Geometry: see drawing. Coordinates: mm, zero at the bounding-box minimum. Coordinates: 2 decimals unless noted, no trailing zeros. Loops run counter-clockwise (first coordinate to the right, second up) from the corner with the lowest first, then second, coordinate; pieces in that order, holes last. Notation, with made-up numbers: (-15.75, 59.5) -> (32.25, 59.5) arc R20 cw to (32.25, 63.5) -> close; hole circle Ø2 at (-10, -31.5). An arc over 180 degrees is marked (long way). Answer as a JSON object with one key per item and string values.
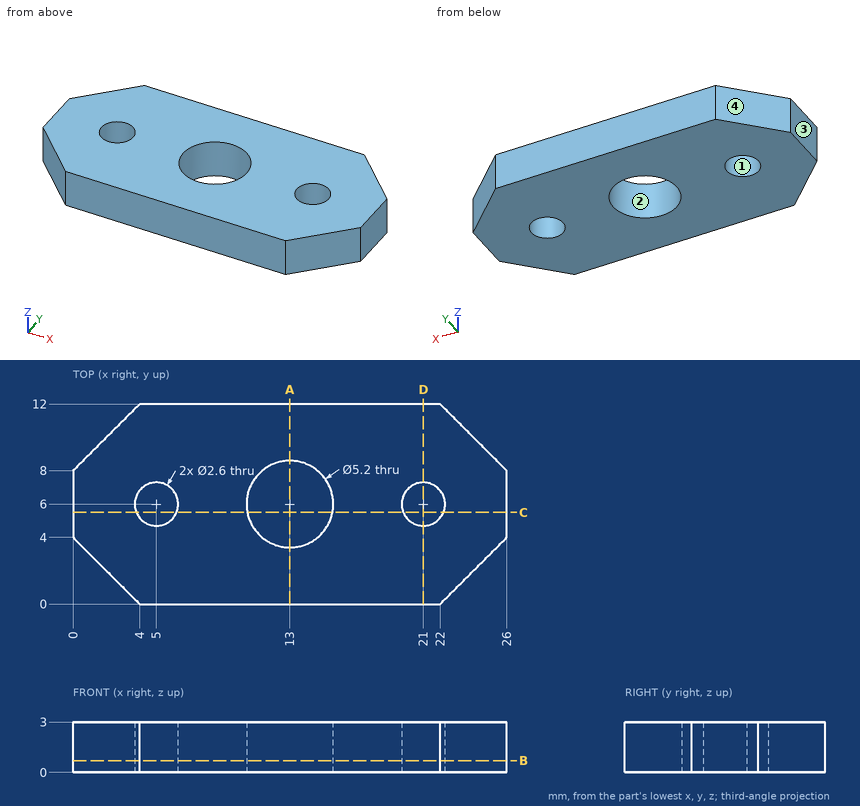
1. Section query A-A (x = 13). Return loops of the section in (y, z), plus the area to 3 significant figures.
Reply:
{"outline": "(0, 0) -> (3.4, 0) -> (3.4, 3) -> (0, 3) -> close; (8.6, 0) -> (12, 0) -> (12, 3) -> (8.6, 3) -> close", "area": "20.4 mm2"}
2. Mould query, pull axis Y, two halves, no side actions, for the marked faces 1, 2, 3 and 4. Classes: pulls with the +Y half, pulls with the -Y half, needs draft (parallel to the pull), parting line crosses it, or undercut.
Reply:
{"face 1": "undercut", "face 2": "undercut", "face 3": "needs draft", "face 4": "pulls with the +Y half"}
3. Section query C-C (y = 5.5). Return loops of the section in (x, z).
Reply:
{"outline": "(0, 0) -> (3.8, 0) -> (3.8, 3) -> (0, 3) -> close; (6.2, 0) -> (10.45, 0) -> (10.45, 3) -> (6.2, 3) -> close; (15.55, 0) -> (19.8, 0) -> (19.8, 3) -> (15.55, 3) -> close; (22.2, 0) -> (26, 0) -> (26, 3) -> (22.2, 3) -> close"}
4. Section query D-D (x = 21). Return loops of the section in (y, z), plus the area to 3 significant figures.
Reply:
{"outline": "(0, 0) -> (4.7, 0) -> (4.7, 3) -> (0, 3) -> close; (7.3, 0) -> (12, 0) -> (12, 3) -> (7.3, 3) -> close", "area": "28.2 mm2"}
5. Section query B-B (z = 0.7). Return loops of the section in (x, y).
Reply:
{"outline": "(0, 4) -> (4, 0) -> (22, 0) -> (26, 4) -> (26, 8) -> (22, 12) -> (4, 12) -> (0, 8) -> close; hole circle Ø2.6 at (5, 6); hole circle Ø5.2 at (13, 6); hole circle Ø2.6 at (21, 6)"}
6. Line query: line 1 along Y through (x, z) = (5, 2); line 2 along X through (y, z) = (6.5, 1.4); line 3 along Y through (x, z) = (13.5, 1.65). Output: solid intervals per line, ascending.
Reply:
{"line 1": "y = 0 to 4.7, 7.3 to 12", "line 2": "x = 0 to 3.8, 6.2 to 10.45, 15.55 to 19.8, 22.2 to 26", "line 3": "y = 0 to 3.45, 8.55 to 12"}
